Source: CAD feature listing. Evaluate the final solid. Frame: model axes, mm. A direction names the side the tool comes from. Give positions to 0.01 mm unless a question says otherwise; leave off trailing zeros. Order: outer loops, then holes, each group sorted by start corner. A loop starts at its lowest first (then second) coordinate and runs counter-clockwise, first axis right, second up. Notation, with made-up numbers: (60, 26) - (65, 26) arc R36 ccw to (65, 62) - close; hole circle Ø1 at (17, 58.25). An arc over 180 degrees is marked (long way). One line per item, written item: value. Start each with the question number.
from build123d import *

# Parameters (mm, degrees)
F0_W     = 86
F0_H     = 51
F0_W_2   = 80
F0_H_2   = 45
F0_R     = 1.5
F1_DEPTH = 3
F2_DEPTH = 15
F3_W     = 3
F3_H     = 16
F4_DEPTH = 10
F6_R     = 1.5
F7_DEPTH = 2
F8_R     = 2


with BuildPart() as f1:
    # F0 (on Top) → F1 (new body)
    with BuildSketch(Plane.XY):
        Rectangle(F0_W, F0_H)
        Rectangle(F0_W_2, F0_H_2, mode=Mode.SUBTRACT)
        Rectangle(F0_W_2, F0_H_2)
        with Locations((-35, -19)):
            Circle(F0_R, mode=Mode.SUBTRACT)
        with Locations((35, -19)):
            Circle(F0_R, mode=Mode.SUBTRACT)
        with Locations((-35, 19)):
            Circle(F0_R, mode=Mode.SUBTRACT)
        with Locations((35, 19)):
            Circle(F0_R, mode=Mode.SUBTRACT)
    extrude(amount=F1_DEPTH)

    # F0 (on Top) → F2 (join)
    with BuildSketch(Plane.XY):
        Rectangle(F0_W, F0_H)
        Rectangle(F0_W_2, F0_H_2, mode=Mode.SUBTRACT)
    extrude(amount=F2_DEPTH)

    # F3 (on face) → F4 (cut)
    with BuildSketch(Plane.XY.offset(15)):
        with Locations((-41.5, 0)):
            Rectangle(F3_W, F3_H)
        with Locations((41.5, 0)):
            Rectangle(F3_W, F3_H)
    extrude(amount=-F4_DEPTH, mode=Mode.SUBTRACT)

    # F6 (on face) → F7 (cut)
    with BuildSketch(Plane(origin=(0, 0, 0), x_dir=(1, 0, 0), z_dir=(0, 0, -1))):
        Polygon((-34.1939000371, 15.9285937776), (-31.9370342046, 18.1623999346), (-32.7431341675, 21.2338061571), (-35.8060999629, 22.0714062224), (-38.0629657954, 19.8376000654), (-37.2568658325, 16.7661938429), align=None)
        with Locations((-35, 19)):
            Circle(F6_R, mode=Mode.SUBTRACT)
        Polygon((-33.8121897672, -21.9449007087), (-31.8557360582, -19.4437765179), (-33.043546291, -16.4988758092), (-36.1878102328, -16.0550992913), (-38.1442639418, -18.5562234821), (-36.956453709, -21.5011241908), align=None)
        with Locations((-35, -19)):
            Circle(F6_R, mode=Mode.SUBTRACT)
        Polygon((35.6810371117, -22.1015353917), (38.0265269958, -19.9609722562), (37.3454898841, -16.8594368645), (34.3189628883, -15.8984646083), (31.9734730042, -18.0390277438), (32.6545101159, -21.1405631355), align=None)
        with Locations((35, -19)):
            Circle(F6_R, mode=Mode.SUBTRACT)
        Polygon((35.0691377179, 15.8253262673), (37.7839169602, 17.4725381537), (37.7147792423, 20.6472118864), (34.9308622821, 22.1746737327), (32.2160830398, 20.5274618463), (32.2852207577, 17.3527881136), align=None)
        with Locations((35, 19)):
            Circle(F6_R, mode=Mode.SUBTRACT)
    extrude(amount=-F7_DEPTH, mode=Mode.SUBTRACT)

    # F8
    f8_edges = [f1.edges().sort_by_distance(p)[0] for p in [
        (0, -25.5, 15),
        (0, 25.5, 15),
        (43, 16.75, 15),
        (43, -16.75, 15),
        (-43, 16.75, 15),
        (-43, -16.75, 15),
    ]]
    fillet(f8_edges, radius=F8_R)


solid = f1.part
1. Section D-D on y = -19. Return the cut outline in (x, z).
2. Section A-A on z = 10. Return the cut outline in (x, y), then the cut area to 3 significant figures.
3. Section C-C on y = 11. Return the cut outline in (x, z), then the cut area to 3 significant figures.
4. Set-up query: faces 4 (the flat face through (-1, 22.5, 9)), 5 (the flat face through (-42, -8, 10)), 6 (the flat face through (-35.41, 21.72, 0.99)). Return all of +Z, -Z, +X, -X, +Y, -Y with unobstructed straight access to the full face (end or side cutting, diameter ignored); none if empty.
5. Section B-B on x = 9. Return the cut outline in (y, z), then the cut area to 3 significant figures.
6. Ray query, L1, parallel to X at y = -19, z = 2.55; L2, parallel to Y at x = 35, z = 2.5; L3, parallel to Y at x = 9, z = 9.25. Return the intervals inside material, ascending.
7. Contact query for flat-ended pins moving along their axis: pin 1 Ø3.5 at (x, y) = (-35, 19) entering from -Z; pin 2 Ø3.5 at (x, y) = (35, -19) entering from +Z; pin 3 Ø1.5 at (x, y) = (-41.5, 3) entering from +Z. Output: stop coordinate, or through.
8. Draft query along Y for faces 1 (the flat face through (-32.44, 17.99, 0.99)), 2 (the flat face through (-1, -25.5, 6)), 3 (the cylindrical face through (42.4, 16.87, 14.43)). Return one class per face: pulls with the +Y half, pulls with the -Y half, needs draft (parallel to the pull), parting line crosses it, or undercut.
Data:
1. outline: (-43, 0) - (-37.84, 0) - (-37.84, 2) - (-36.5, 2) - (-36.5, 3) - (-40, 3) - (-40, 15) - (-41, 15) arc R2 ccw to (-43, 13) - close; (-33.5, 2) - (-32.16, 2) - (-32.16, 0) - (32.25, 0) - (32.25, 2) - (33.5, 2) - (33.5, 3) - (-33.5, 3) - close; (36.5, 2) - (37.75, 2) - (37.75, 0) - (43, 0) - (43, 13) arc R2 ccw to (41, 15) - (40, 15) - (40, 3) - (36.5, 3) - close
2. outline: (-43, -25.5) - (43, -25.5) - (43, -8) - (40, -8) - (40, -22.5) - (-40, -22.5) - (-40, -8) - (-43, -8) - close; (-43, 8) - (-40, 8) - (-40, 22.5) - (40, 22.5) - (40, 8) - (43, 8) - (43, 25.5) - (-43, 25.5) - close
2. area: 690 mm2
3. outline: (-43, 0) - (43, 0) - (43, 13) arc R2 ccw to (41, 15) - (40, 15) - (40, 3) - (-40, 3) - (-40, 15) - (-41, 15) arc R2 ccw to (-43, 13) - close
3. area: 328 mm2
4. face 4: +Z
4. face 5: +Z, +X, -X
4. face 6: -Z
5. outline: (-25.5, 0) - (25.5, 0) - (25.5, 13) arc R2 ccw to (23.5, 15) - (22.5, 15) - (22.5, 3) - (-22.5, 3) - (-22.5, 15) - (-23.5, 15) arc R2 ccw to (-25.5, 13) - close
5. area: 223 mm2
6. L1: x = -43 to -36.5, -33.5 to 33.5, 36.5 to 43
6. L2: y = -25.5 to -20.5, -17.5 to 17.5, 20.5 to 25.5
6. L3: y = -25.5 to -22.5, 22.5 to 25.5
7. pin 1: stops at z = 2
7. pin 2: stops at z = 3
7. pin 3: stops at z = 5
8. face 1: undercut
8. face 2: pulls with the -Y half
8. face 3: needs draft
